Geometry check sheet. Reference: drawing and pictorial views, mm from the part's lowest x, y, z. A direction names the side the tool comes from. Give positions to 0.01 mm unless a question says otherwise; leave off trailing zeros. Order: outer loops, then holes, each group sorted by start corner. A loop starts at its lowest first (then second) coordinate and runs counter-clockwise, first axis right, second up.
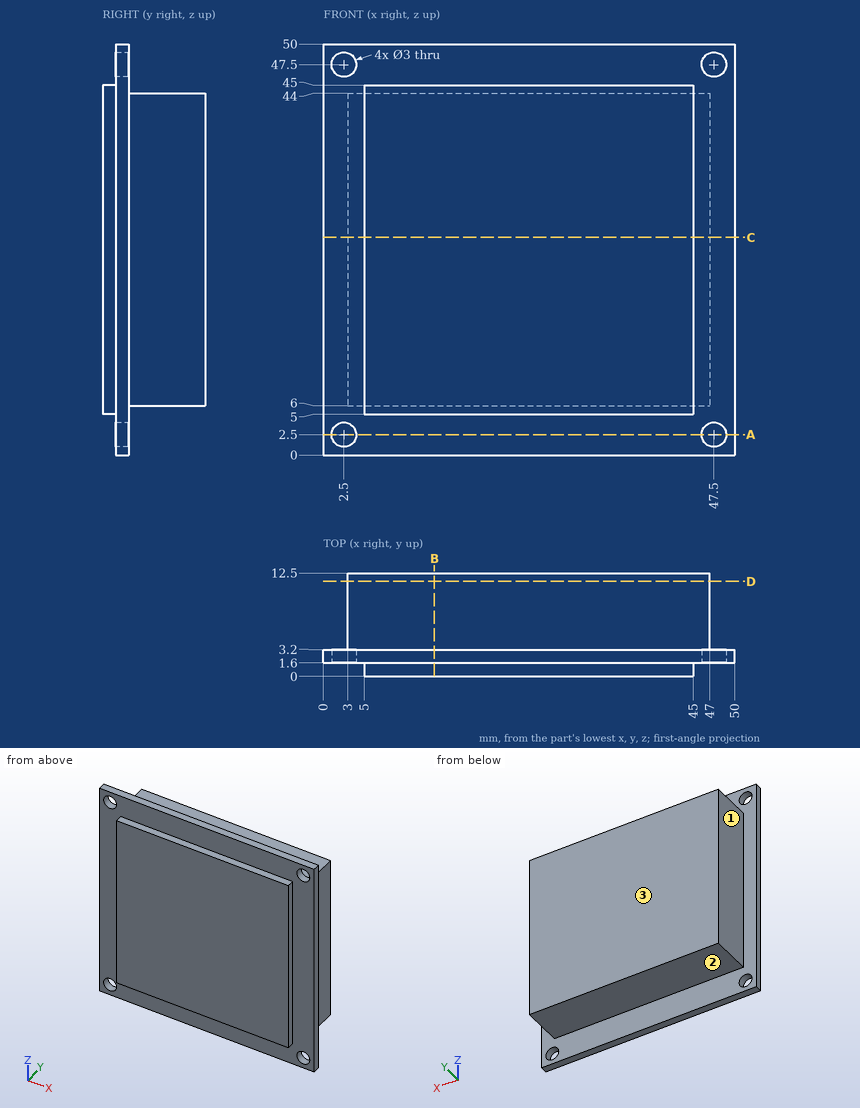
(1) Cross-section at B-B on x = 13.5. Enter the section's corners in (y, z), then the cut area to 3 significant figures.
Response values:
outline: (0, 5) - (1.6, 5) - (1.6, 0) - (3.2, 0) - (3.2, 6) - (12.5, 6) - (12.5, 44) - (3.2, 44) - (3.2, 50) - (1.6, 50) - (1.6, 45) - (0, 45) - close
area: 497 mm2
(2) Cross-section at D-D on y = 11.5. Enter the section's corners in (x, z), then the cut area to 3 significant figures.
Response values:
outline: (3, 6) - (47, 6) - (47, 44) - (3, 44) - close
area: 1,670 mm2
(3) Set-up check for the marked faces 1, 2 and 3: record each of +Z, -Z, +X, -X, +Y, -Y from which the full face is reachable in a straight line by a thin tool's end or side.
Response values:
face 1: +Z, -Z, -X, +Y
face 2: -Z, +X, -X, +Y
face 3: +Z, -Z, +X, -X, +Y
(4) Material ranges on L1, parallel to X at y = 2.8, z = 47.5; L2, parallel to Z at x = 19.5, y = 12; L3, parallel to X at y = 7.5, z = 22, recorded low to high.
Response values:
L1: x = 0 to 1, 4 to 46, 49 to 50
L2: z = 6 to 44
L3: x = 3 to 47
(5) Gauge pin test, flat ends, axial feed: pin 1 Ø6 at (x, y) = (18, 10) entering from -Z; pin 2 Ø1 at (y, z) = (10, 32) entering from -X; pin 3 Ø4.5 at (y, z) = (7, 20) entering from +X; pin 4 Ø1.8 at (x, z) = (2.5, 47.5) entering from -Y. Record the tip position at first contact, or that the pin passes through.
Response values:
pin 1: stops at z = 6
pin 2: stops at x = 3
pin 3: stops at x = 47
pin 4: passes through
(6) Cross-section at A-A on z = 2.5. Enter the section's corners in (x, y), then the cut area to 3 significant figures.
Response values:
outline: (0, 1.6) - (1, 1.6) - (1, 3.2) - (0, 3.2) - close; (4, 1.6) - (46, 1.6) - (46, 3.2) - (4, 3.2) - close; (49, 1.6) - (50, 1.6) - (50, 3.2) - (49, 3.2) - close
area: 70.4 mm2
(7) Cross-section at C-C on z = 26.5. Enter the section's corners in (x, y), then the cut area to 3 significant figures.
Response values:
outline: (0, 1.6) - (5, 1.6) - (5, 0) - (45, 0) - (45, 1.6) - (50, 1.6) - (50, 3.2) - (47, 3.2) - (47, 12.5) - (3, 12.5) - (3, 3.2) - (0, 3.2) - close
area: 553 mm2
